from build123d import *

# Parameters (mm, degrees)
ODEBRAT_VYSUNUT_M1_REACH = 17.125
ODEBRAT_VYSUNUT_M2_REACH = 17.125
KRUHOV_POLE1_COUNT       = 9


with BuildPart() as part:
    # Skica1 → Otočit kolem osy1 (revolve)
    with BuildSketch(Plane.XY):
        Polygon((0, 0), (0, 6.75), (-1.876388375, 10), (-1.010362971, 10.5), (1, 7.017949192), (1, 0), align=None)
    revolve(axis=Axis((0, 0, 0), (-1, 0, 0)))

    # Skica2 → Odebrat vysunutím1 (cut, up to next)
    with BuildSketch(Plane(origin=(1, 0, 0), x_dir=(0, 0, -1), z_dir=(1, 0, 0)), mode=Mode.PRIVATE) as odebrat_vysunut_m1_sk1:
        with BuildLine():
            Line((1.5, -4.769696007), (1.5, -3.5))
            Line((1.5, -3.5), (-1.5, -3.5))
            Line((-1.5, -3.5), (-1.5, -4.769696007))
            ThreePointArc((-1.5, -4.769696007), (0, 5), (1.5, -4.769696007))
        make_face()
    odebrat_vysunut_m1_tool1 = extrude(odebrat_vysunut_m1_sk1.sketch, amount=-ODEBRAT_VYSUNUT_M1_REACH, mode=Mode.PRIVATE) & part.part
    add(odebrat_vysunut_m1_tool1.solids().sort_by_distance((1, 0.242366, 0))[0], mode=Mode.SUBTRACT)

    # Skica3 → Odebrat vysunutím2 (cut, up to next)
    with BuildSketch(Plane(origin=(1, 0, 0), x_dir=(0, 0, -1), z_dir=(1, 0, 0)), mode=Mode.PRIVATE) as odebrat_vysunut_m2_sk1:
        with BuildLine():
            Line((-1.5, -10.392304845), (-1.5, -8.366600265))
            ThreePointArc((-1.5, -8.366600265), (-2.907171218, -7.987387277), (-4.228880321, -7.373369056))
            Line((-4.228880321, -7.373369056), (-5.530978126, -8.925148793))
            ThreePointArc((-5.530978126, -8.925148793), (-3.591211505, -9.866772518), (-1.5, -10.392304845))
        make_face()
    odebrat_vysunut_m2_tool1 = extrude(odebrat_vysunut_m2_sk1.sketch, amount=-ODEBRAT_VYSUNUT_M2_REACH, mode=Mode.PRIVATE) & part.part
    odebrat_vysunut_m2 = odebrat_vysunut_m2_tool1.solids().sort_by_distance((1, -8.932717, 3.251243))[0]
    add(odebrat_vysunut_m2, mode=Mode.SUBTRACT)

    # Kruhové pole1: Odebrat vysunutím2 ×9 about axis
    kruhov_pole1_axis = Axis((0, 0, 0), (1, 0, 0))
    for i in range(1, KRUHOV_POLE1_COUNT):
        add(odebrat_vysunut_m2.rotate(kruhov_pole1_axis, i * 360 / KRUHOV_POLE1_COUNT), mode=Mode.SUBTRACT)


solid = part.part
CAD build for the part. Positions are in the model's coordinates, mm. A direction names the side the tool comes from. Coordinates: 2 decimals unless noted, no trailing zeros. Order: outer loops, then holes, each group sorted by start corner. A loop starts at its lowest first (then second) coordinate and runs counter-clockwise, first axis right, second up.
Item 1: Band-saw the part on B-B on x = 0.7. List the corners of the cut face in (y, z), plus the area to 3 significant figures.
Check sheet entries:
outline: circle Ø15.08 at (0, 0); hole (-4.77, -1.5) arc R5 ccw (long way) to (-4.77, 1.5) - (-3.5, 1.5) - (-3.5, -1.5) - close
area: 104 mm2
Item 2: Pin check, flat tips, straight feed: pin 1 Ø5 at (y, z) = (0.5, -5.5) entering from -X; pin 2 Ø1.1 at (x, y) = (0.5, -4.5) entering from -Z; pin 3 Ø6 at (y, z) = (-3, 6) entering from -X; pin 4 Ø4 at (y, z) = (0.5, 2.5) entering from -X. Stop position of each tip, or through.
Check sheet entries:
pin 1: stops at x = -0.73
pin 2: stops at z = -7.46
pin 3: stops at x = -1.6
pin 4: passes through
Item 3: Drill centre lines: L1, parallel to Y at x = -0.3, z = -5.25; L2, parallel to Y at x = 0.6, z = 0; L3, parallel to Z at x = 0.75, y = 0. Where is each one in solid material? Low to high.
Check sheet entries:
L1: y = -7.64 to -5.03, 5.03 to 6.68
L2: y = -7.71 to -3.5, 5 to 7.71
L3: z = -7.45 to -5, 5 to 7.45
Item 4: Band-saw the part on A-A on z = 0. List the corners of the cut face in (x, y).
Check sheet entries:
outline: (-1.88, -10) - (-1.01, -10.5) - (1, -7.02) - (1, -3.5) - (0, -3.5) - (0, -6.75) - close; (-1.01, 8.5) - (0, 6.75) - (0, 5) - (1, 5) - (1, 7.02) - (0.14, 8.5) - close
Item 5: Two-plate mould, pull along Y, no slides. Class faces 5 (the face through (-0.425, -4.232, -7.371)), 6 (the face through (-0.85, 5.87, -7.17)), 7 (the face through (-1.437, -7.841, -6.607)): +Y half, -Y half, draft (parallel to the pull), parting line (faces both ways), or undercut.
Check sheet entries:
face 5: undercut
face 6: +Y half
face 7: -Y half
Item 6: 3-axis set-ups, long thin cutter, end or side, ignore diameter. For faces 1 (the face through (-0.852, -0.115, 9.29)), 2 (the face through (-0.85, -0.11, -9.26)), 3 (the face through (-0.852, 9.129, 1.726)), 4 (the face through (-0.852, -3.064, 8.741)): which of +Z, -Z, +X, -X, +Y, -Y reach the whole face in a straight line?
Check sheet entries:
face 1: +Z, +X, -X
face 2: -Z, +X, -X
face 3: +X, -X, +Y
face 4: +X, -X, -Y
